Autodesk Inventor part; units mm, degrees
ref_plane "YZ Plane" through (0, 0, 0) normal (1, 0, 0) x (0, 1, 0)
ref_plane "XZ Plane" through (0, 0, 0) normal (0, 1, 0) x (-1, 0, 0)
ref_plane "XY Plane" through (0, 0, 0) normal (0, 0, 1) x (1, 0, 0)
sketch "Sketch1" plane through (0, 0, 0) normal (0, 0, 1) x (1, 0, 0)
  arc A0 (6.0118, 7.7827) -> (6.4404, 9.2521) centre (8, 8) ccw construction
  arc A1 (7.7827, -6.0118) -> (9.2521, -6.4404) centre (8, -8) ccw construction
  circle A2 centre (8, 8) radius 1.9939 construction
  circle A3 centre (8, -8) radius 1.9939 construction
  line L0 (6.0061, 8) -> (6.0061, -8) construction
  line L1 (1.9277, 2.1329) -> (2.8194, -0.5629) construction
  arc A4 (1.9277, 2.1329) -> (2.8194, -0.5629) centre (0, 0) ccw construction
  line L2 (9.9939, 8) -> (6.0061, 8) construction
  line L3 (6.0061, 8) -> (6.0061, -8) construction
  line L4 (6.0061, -8) -> (9.9939, -8) construction
  line L5 (9.9939, -8) -> (9.9939, 8) construction
  arc A5 (12.7621, 7.9367) -> (3.2375, 8) centre (8, 8) ccw construction
  line L6 (8, 8) -> (3.2375, 8) construction
  line L7 (8, 8) -> (12.7625, 8) construction
  line L8 (12.7625, 10.7686) -> (3.2375, 10.7686) construction
  line L9 (3.2375, 10.7686) -> (3.2375, -14.5363) construction
  line L10 (3.2375, -10.7686) -> (12.7625, -10.7686) construction
  line L11 (12.7625, -11.6614) -> (12.7625, 10.7686) construction
  line L12 (12.7625, 8) -> (12.7625, -11.6614) construction
  line L13 (3.2375, 8) -> (3.2375, -14.5363) construction
  line L14 (125.2938, -2.5112) -> (119.3124, -4.6433) construction
  line L15 (120.3686, -7.6063) -> (119.3124, -4.6433) construction
  circle A6 centre (64.263, -105.1393) radius 2 construction
  circle A7 centre (0, 0) radius 1.9939 construction
  line L16 (64.263, -105.1393) -> (0, 0) construction
  line L17 (0, 0) -> (-1.7037, -1.0359) construction
  line L18 (0, 0) -> (1.9939, 0) construction
  line L19 (0, 0) -> (1.7037, 1.0359) construction
  line L20 (64.263, -105.1393) -> (62.5541, -106.1783) construction
  line L21 (64.263, -105.1393) -> (66.263, -105.1393) construction
  line L22 (64.263, -105.1393) -> (65.9719, -104.1002) construction
  line L23 (1.7037, 1.0359) -> (65.9719, -104.1002) construction
  line L24 (65.9719, -104.1002) -> (62.5591, -106.1865) construction
  line L25 (62.5591, -106.1865) -> (-1.7091, -1.0504) construction
  line L26 (-1.7091, -1.0504) -> (1.7037, 1.0359) construction
  line L27 (-5.5766, -0.1174) -> (61.6261, -110.0539) construction
  line L28 (61.6261, -110.0539) -> (69.8394, -105.0332) construction
  line L29 (69.8394, -105.0332) -> (0.7437, 8) construction
  line L30 (2.6367, 4.9033) -> (-5.5766, -0.1174) construction
  line L31 (64.263, -105.1393) -> (68.3721, -102.633) construction
  line L32 (12.7625, -11.6614) -> (68.3721, -102.633) construction
  line L33 (64.263, -105.1393) -> (60.1589, -107.6537) construction
  line L34 (68.3721, -102.633) -> (60.1589, -107.6537) construction
  line L35 (60.1589, -107.6537) -> (3.2375, -14.5363) construction
  arc A8 (25.7824, -64.2706) -> (22.8, -65.3296) centre (24.3335, -64.9192) ccw construction
  circle A9 centre (43.9887, -120.2705) radius 1.5 construction
  circle A10 centre (43.9887, -120.2705) radius 60.325 construction
  circle A11 centre (34.3115, -56.1364) radius 1.778 construction
  circle A12 centre (8, 8) radius 4.7625
  line L36 (12.7625, -11.6614) -> (3.2375, -14.5363)
  line L37 (3.2375, -14.5363) -> (60.1589, -107.6537)
  line L38 (60.1589, -107.6537) -> (68.3721, -102.633)
  line L39 (68.3721, -102.633) -> (12.7625, -11.6614)
  circle A13 centre (34.3115, -56.1364) radius 1.778
  circle A14 centre (13.9136, -22.7595) radius 1.778
  circle A15 centre (19.013, -31.1037) radius 1.778
  circle A16 centre (24.1123, -39.4479) radius 1.778
  circle A17 centre (29.2117, -47.7921) radius 1.778
  circle A18 centre (39.4103, -64.4804) radius 1.778
  circle A19 centre (44.5097, -72.8246) radius 1.778
  circle A20 centre (49.609, -81.1688) radius 1.778
  circle A21 centre (54.7084, -89.513) radius 1.778
  circle A22 centre (8, -8) radius 1.9939
  circle A23 centre (8, 8) radius 1.9939
  point P0 (0, 0)
  dimension "d1" = 3.9878
  dimension "d0" = 3.9878
  dimension "d3" = 4.7625
  dimension "d4" = 180
  dimension "d5" = 2.7686
  dimension "d6" = 3.9878
  dimension "d7" = 148.7
  dimension "d8" = 148.7
  dimension "d9" = 2.8131
  dimension "d11" = 3.556
  dimension "d98" = 3.9878
  dimension "d99" = 3.9878
extrude "Extrusion1" add sketch "Sketch1" along normal blind 3.175 contours A12 | A23
ref_plane "Work Plane1" through (0, 0, 0) normal (0, 0, 1) x (1, 0, 0)
sketch "Sketch2" plane through (0, 0, 0) normal (0, 0, 1) x (1, 0, 0)
  circle A0 centre (8, 8) radius 4.7625
  line L0 (12.7625, 8) -> (3.2375, 8)
  line L1 (3.2375, 8) -> (3.2375, -14.5363)
  line L2 (3.2375, -14.5363) -> (12.7625, -14.5363)
  line L3 (12.7625, -14.5363) -> (12.7625, 8)
  line L4 (3.2375, -14.5363) -> (60.325, -107.95)
  line L5 (60.325, -107.95) -> (68.4525, -102.9831)
  line L6 (68.4525, -102.9831) -> (11.365, -9.5694)
  line L7 (11.365, -9.5694) -> (3.2375, -14.5363)
  point P0 (0, 0)
  dimension "d14" = 9.525
extrude "Extrusion2" add sketch "Sketch2" along normal blind 3.175 contours L3 L6 L7 L1 A0 | A0 L0 | L6 L5 L4 L2 L3 | L3 L2 L7 L6 picked at (6.8117, 6.9473)
hole "Hole1" at (34.311, -56.1362, 0) direction (0, 0, 1) diameter 3.556 end through all
hole "Hole2" at (49.6089, -81.1686, 0) direction (0, 0, 1) diameter 3.556 end through all
hole "Hole3" at (44.509, -72.8243, 0) direction (0, 0, 1) diameter 3.556 end through all
hole "Hole4" at (54.7081, -89.5129, 0) direction (0, 0, 1) diameter 3.556 end through all
hole "Hole5" at (39.4103, -64.4805, 0) direction (0, 0, 1) diameter 3.556 end through all
hole "Hole6" at (29.2063, -47.787, 0) direction (0, 0, 1) diameter 3.556 end through all
hole "Hole7" at (24.11, -39.4457, 0) direction (0, 0, 1) diameter 3.556 end through all
hole "Hole8" at (19.0131, -31.1028, 0) direction (0, 0, 1) diameter 3.556 end through all
hole "Hole9" at (13.917, -22.7563, 0) direction (0, 0, 1) diameter 3.556 end through all
sketch "Sketch3" plane through (60.325, -107.95, 0) normal (-0.8533, -0.5215, 0) x (0, 0, 1)
  point P0 (0, 123.5682)
sketch "Sketch4" plane through (0, 0, 3.175) normal (0, 0, 1) x (1, 0, 0)
  spline S0 degree 3 poles (-25.2788, -2.0557) (-25.3112, -1.9605) (-25.3341, -1.8916) (-25.3588, -1.8128) (-25.3613, -1.8009) (-25.3441, -1.8374) (-25.3155, -1.9119) (-25.2521, -2.0803) (-25.2004, -2.2209) (-25.0761, -2.5633) (-25.0055, -2.7599) (-24.8596, -3.169) (-24.7792, -3.3953) (-24.6138, -3.8659) (-24.5358, -4.0898) (-24.3927, -4.5052) (-24.3289, -4.6925) (-24.2382, -4.9635) (-24.1921, -5.103) (-24.1408, -5.2711) (-24.1321, -5.3068) (-24.1428, -5.2998) (-24.1636, -5.2531) (-24.2396, -5.0631) (-24.2901, -4.9305) (-24.3621, -4.7401) (-24.4003, -4.6379) (-24.4829, -4.4155) (-24.5269, -4.296) (-24.5725, -4.1714) knots 0.000001 0.000001 0.000001 0.000001 0.060915 0.060915 0.118968 0.118968 0.203575 0.203575 0.324675 0.324675 0.441995 0.441995 0.548902 0.548902 0.648718 0.648718 0.748605 0.748605 0.82225 0.82225 0.878767 0.878767 0.938156 0.938156 1.008318 1.008318 1.073219 1.073219 1.138691 1.138691 1.138691 1.138691
  point P0 (0, 0)
sketch "Sketch5" plane through (0, 0, 0) normal (0, 0, -1) x (-1, 0, 0)
  arc A0 (-9.9544, 7.5753) -> (-9.6822, 9.0817) centre (-8, 8) ccw
  arc A1 (-7.5753, -9.9544) -> (-9.0817, -9.6822) centre (-8, -8) ccw
  circle A2 centre (-8, 8) radius 2
  circle A3 centre (-8, -8) radius 2
  point P0 (0, 0)
hole "Hole10" at (8, -8, 0) direction (0, 0, 1) diameter 3.9878 end through all
hole "Hole11" at (8, 8, 0) direction (0, 0, 1) diameter 3.9878 end through all
sketch "Sketch6" plane through (0, 0, 3.175) normal (0, 0, 1) x (1, 0, 0)
  point P0 (0, 0)
sketch "Sketch7" plane through (0, 0, 3.175) normal (0, 0, 1) x (1, 0, 0)
  circle A0 centre (19.0131, -31.1028) radius 1.778 construction
  circle A1 centre (13.917, -22.7563) radius 1.778 construction
  line L0 (19.0131, -31.1028) -> (13.917, -22.7563) construction
  point P0 (0, 0)
properties part number "CollectorArmWithAngle"
Read the model definition and answer for the solid it produces. Units are mm, in the model's axes. A direction names the side the tool comes from. Give positions to 0.01 mm unless a question says otherwise; leave off trailing zeros. Loops run counter-clockwise (first coordinate to the right, second up) from the corner with the lowest first, then second, coordinate; pieces in that order, holes last.
Item 1: For faces 1 (the cylindrical face through (30.288, -49.198, 1.61)), 2 (the flat face through (12.762, -2, 2)), determine the directions among +Z, -Z, +X, -X, +Y, -Y from which every point of the face is accessible in a straight line to the end or side of a thin tool.
Item 2: The mould has two halves that part along X. Classify faces 3 (the flat face through (64.332, -105.501, 1.565)), 4 (the cylindrical face through (24.03, -41.22, 1.61)), 5 (the flat face through (33, -47, 0)), 6 (the flat face through (31.38, -60.59, 1.57)): released by +X, released by -X, zero draft, split by the parting line, or undercut.
Item 3: The part is cut by section D-D (x = 24.11). Write down the section's boundary in (y, z) (1 decimal).
Item 4: Each of these flat-tipped pins is pushed along its axis until it touches: pin 1 Ø1 at (x, z) = (43.5, 2.5) entering from -Y; pin 2 Ø1.6 at (y, z) = (2.5, 1.5) entering from +X. Where does it stop, or does it pass through?
Item 5: The part is cut by section C-C (x = 8). Write down the section's boundary in (y, z) (1 decimal).
Item 6: Find the intervals of material crossed by line 1 along X through (y, z) = (-8, 1.75); line 2 along Y through (x, z) = (8, 1.7); line 3 along X through (y, z) = (-73.5, 0.7), in increasing order.
Item 7: The part is cut by section B-B (z = 2.2). Give the number of separate pieces and of enclosed holes in the cut face, and give its area (3 significant figures).
Item 8: The part is cut by section A-A (y = -8). Write down the section's boundary in (x, z) (1 decimal), and give its area (3 significant figures).
Taken from the geometry:
1. face 1: +Z, -Z
1. face 2: +Z, -Z, +X, +Y
2. face 3: released by +X
2. face 4: undercut
2. face 5: zero draft
2. face 6: released by -X
3. outline: (-48.7, 0) - (-41.2, 0) - (-41.2, 3.2) - (-48.7, 3.2) - close; (-37.7, 0) - (-30.4, 0) - (-30.4, 3.2) - (-37.7, 3.2) - close
4. pin 1: stops at y = -81.24
4. pin 2: stops at x = 12.76
5. outline: (-22.3, 0) - (-10, 0) - (-10, 3.2) - (-22.3, 3.2) - close; (-6, 0) - (6, 0) - (6, 3.2) - (-6, 3.2) - close; (10, 0) - (12.8, 0) - (12.8, 3.2) - (10, 3.2) - close
6. line 1: x = 3.24 to 6.01, 9.99 to 12.76
6. line 2: y = -22.33 to -9.99, -6.01 to 6.01, 9.99 to 12.76
6. line 3: x = 39.27 to 42.86, 46.15 to 50.43
7. separate pieces: 1
7. enclosed holes: 11
7. area: 1,150 mm2
8. outline: (3.2, 0) - (6, 0) - (6, 3.2) - (3.2, 3.2) - close; (10, 0) - (12.8, 0) - (12.8, 3.2) - (10, 3.2) - close
8. area: 17.6 mm2
